Work out the finished part from the listing and answer in its coordinate system (mm). Face numbers are marked on the shaded views. A direction names the side the tool comes from. Give positions to 0.01 mm unless a question says otherwise; leave off trailing zeros. Write each loop counter-clockwise with the first axis right and the second up, starting at its lowest first coordinate (ties: lowest second). Pieces come first, ordered by that corner, then holes. Notation, with made-up numbers: (2.25, -23) - (56.25, -23) arc R25 cw to (56.25, 4) - close; hole circle Ø6 at (72, 22). An arc over 180 degrees is marked (long way). Write item = value, one per line.
from build123d import *

# Parameters (mm, degrees)
SKETCH_1_W          = 110
SKETCH_1_H          = 52.5
EXTRUDE_1_DEPTH     = 2
SKETCH_2_W          = 110
SKETCH_2_H          = 52.5
SKETCH_2_W_2        = 101.5
SKETCH_2_H_2        = 46.5
EXTRUDE_2_DEPTH     = 8.5
CUT_EXTRUDE_1_DEPTH = 3
SKETCH_5_W          = 8
SKETCH_5_H          = 46.5
CUT_EXTRUDE_2_DEPTH = 3
SKETCH_6_W          = 7
SKETCH_6_H          = 20
SKETCH_6_R          = 1.6
EXTRUDE_3_DEPTH     = 5
CHAMFER_1_SIZE      = 2


with BuildPart() as part:
    # 草图1 → 凸台-拉伸1 (new body)
    with BuildSketch(Plane.XY):
        with Locations((55, 26.25)):
            Rectangle(SKETCH_1_W, SKETCH_1_H)
    extrude(amount=EXTRUDE_1_DEPTH)

    # 草图2 → 凸台-拉伸2 (add)
    with BuildSketch(Plane.XY.offset(2)):
        with Locations((55, 26.25)):
            Rectangle(SKETCH_2_W, SKETCH_2_H)
        with Locations((55, 27.5)):
            Rectangle(SKETCH_2_W_2, SKETCH_2_H_2, mode=Mode.SUBTRACT)
    extrude(amount=EXTRUDE_2_DEPTH)

    # 草图3 → 切除-拉伸1 (cut, through all)
    with BuildSketch(Plane.XY.offset(2)):
        with BuildLine():
            Line((21.166500495, 10.551667335), (28.937295815, 6.991647804))
            ThreePointArc((28.937295815, 6.991647804), (29.429930809, 5.66601182), (28.104294825, 5.173376826))
            Line((28.104294825, 5.173376826), (20.333499505, 8.733396357))
            ThreePointArc((20.333499505, 8.733396357), (19.840864511, 10.059032341), (21.166500495, 10.551667335))
        make_face()
        with BuildLine():
            Line((91.499535297, 49.826623174), (102.166500495, 44.939786901))
            ThreePointArc((102.166500495, 44.939786901), (102.659135489, 43.614150917), (101.333499505, 43.121515923))
            Line((101.333499505, 43.121515923), (90.666534307, 48.008352196))
            ThreePointArc((90.666534307, 48.008352196), (90.173899313, 49.33398818), (91.499535297, 49.826623174))
        make_face()
        with BuildLine():
            Line((21.166500495, 16.051397639), (40.942083467, 6.991647804))
            ThreePointArc((40.942083467, 6.991647804), (41.434718462, 5.66601182), (40.109082477, 5.173376826))
            Line((40.109082477, 5.173376826), (20.333499505, 14.233126661))
            ThreePointArc((20.333499505, 14.233126661), (19.840864511, 15.558762645), (21.166500495, 16.051397639))
        make_face()
        with BuildLine():
            Line((21.166500495, 21.551127943), (52.94687112, 6.991647804))
            ThreePointArc((52.94687112, 6.991647804), (53.439506114, 5.66601182), (52.11387013, 5.173376826))
            Line((52.11387013, 5.173376826), (20.333499505, 19.732856965))
            ThreePointArc((20.333499505, 19.732856965), (19.840864511, 21.058492949), (21.166500495, 21.551127943))
        make_face()
        with BuildLine():
            Line((21.166500495, 32.550588551), (76.956446425, 6.991647804))
            ThreePointArc((76.956446425, 6.991647804), (77.449081419, 5.66601182), (76.123445435, 5.173376826))
            Line((76.123445435, 5.173376826), (20.333499505, 30.732317572))
            ThreePointArc((20.333499505, 30.732317572), (19.840864511, 32.057953556), (21.166500495, 32.550588551))
        make_face()
        with BuildLine():
            Line((21.166500495, 27.050858247), (64.951658772, 6.991647804))
            ThreePointArc((64.951658772, 6.991647804), (65.444293766, 5.66601182), (64.118657782, 5.173376826))
            Line((64.118657782, 5.173376826), (20.333499505, 25.232587268))
            ThreePointArc((20.333499505, 25.232587268), (19.840864511, 26.558223253), (21.166500495, 27.050858247))
        make_face()
        with BuildLine():
            Line((21.166500495, 38.050318854), (88.961234077, 6.991647804))
            ThreePointArc((88.961234077, 6.991647804), (89.453869071, 5.66601182), (88.128233087, 5.173376826))
            Line((88.128233087, 5.173376826), (20.333499505, 36.232047876))
            ThreePointArc((20.333499505, 36.232047876), (19.840864511, 37.55768386), (21.166500495, 38.050318854))
        make_face()
        with BuildLine():
            Line((21.166500495, 43.550049158), (100.96602173, 6.991647804))
            ThreePointArc((100.96602173, 6.991647804), (101.458656724, 5.66601182), (100.13302074, 5.173376826))
            Line((100.13302074, 5.173376826), (20.333499505, 41.73177818))
            ThreePointArc((20.333499505, 41.73177818), (19.840864511, 43.057414164), (21.166500495, 43.550049158))
        make_face()
        with BuildLine():
            Line((21.166500495, 49.049779462), (102.166500495, 11.941405078))
            ThreePointArc((102.166500495, 11.941405078), (102.659135489, 10.615769094), (101.333499505, 10.1231341))
            Line((101.333499505, 10.1231341), (20.333499505, 47.231508484))
            ThreePointArc((20.333499505, 47.231508484), (19.840864511, 48.557144468), (21.166500495, 49.049779462))
        make_face()
        with BuildLine():
            Line((31.475597035, 49.826623174), (102.166500495, 17.441135382))
            ThreePointArc((102.166500495, 17.441135382), (102.659135489, 16.115499398), (101.333499505, 15.622864403))
            Line((101.333499505, 15.622864403), (30.642596045, 48.008352196))
            ThreePointArc((30.642596045, 48.008352196), (30.149961051, 49.33398818), (31.475597035, 49.826623174))
        make_face()
        with BuildLine():
            Line((43.480384687, 49.826623174), (102.166500495, 22.940865686))
            ThreePointArc((102.166500495, 22.940865686), (102.659135489, 21.615229701), (101.333499505, 21.122594707))
            Line((101.333499505, 21.122594707), (42.647383697, 48.008352196))
            ThreePointArc((42.647383697, 48.008352196), (42.154748703, 49.33398818), (43.480384687, 49.826623174))
        make_face()
        with BuildLine():
            Line((55.48517234, 49.826623174), (102.166500495, 28.440595989))
            ThreePointArc((102.166500495, 28.440595989), (102.659135489, 27.114960005), (101.333499505, 26.622325011))
            Line((101.333499505, 26.622325011), (54.65217135, 48.008352196))
            ThreePointArc((54.65217135, 48.008352196), (54.159536356, 49.33398818), (55.48517234, 49.826623174))
        make_face()
        with BuildLine():
            Line((67.489959992, 49.826623174), (102.166500495, 33.940326293))
            ThreePointArc((102.166500495, 33.940326293), (102.659135489, 32.614690309), (101.333499505, 32.122055315))
            Line((101.333499505, 32.122055315), (66.656959002, 48.008352196))
            ThreePointArc((66.656959002, 48.008352196), (66.164324008, 49.33398818), (67.489959992, 49.826623174))
        make_face()
        with BuildLine():
            Line((79.494747645, 49.826623174), (102.166500495, 39.440056597))
            ThreePointArc((102.166500495, 39.440056597), (102.659135489, 38.114420613), (101.333499505, 37.621785619))
            Line((101.333499505, 37.621785619), (78.661746655, 48.008352196))
            ThreePointArc((78.661746655, 48.008352196), (78.16911166, 49.33398818), (79.494747645, 49.826623174))
        make_face()
    extrude(amount=-CUT_EXTRUDE_1_DEPTH, mode=Mode.SUBTRACT)

    # 草图5 → 切除-拉伸2 (cut, through all)
    with BuildSketch(Plane.XY.offset(2)):
        with Locations((8.25, 27.5)):
            Rectangle(SKETCH_5_W, SKETCH_5_H)
    extrude(amount=-CUT_EXTRUDE_2_DEPTH, mode=Mode.SUBTRACT)

    # 草图6 → 凸台-拉伸3 (add)
    with BuildSketch(Plane.XY.offset(10.5)):
        with Locations((113.5, 27.5)):
            Rectangle(SKETCH_6_W, SKETCH_6_H)
        with Locations((113.5, 32.5)):
            Circle(SKETCH_6_R, mode=Mode.SUBTRACT)
        with Locations((113.5, 22.5)):
            Circle(SKETCH_6_R, mode=Mode.SUBTRACT)
        with Locations((-3.5, 27.5)):
            Rectangle(SKETCH_6_W, SKETCH_6_H)
        with Locations((-3.5, 22.5)):
            Circle(SKETCH_6_R, mode=Mode.SUBTRACT)
        with Locations((-3.5, 32.5)):
            Circle(SKETCH_6_R, mode=Mode.SUBTRACT)
    extrude(amount=-EXTRUDE_3_DEPTH)

    # 倒角1
    chamfer_1_edges = [part.edges().sort_by_distance(p)[0] for p in [
        (110, 17.5, 8),
        (110, 37.5, 8),
        (117, 37.5, 8),
        (117, 17.5, 8),
        (0, 37.5, 8),
        (0, 17.5, 8),
        (-7, 17.5, 8),
        (-7, 37.5, 8),
    ]]
    chamfer(chamfer_1_edges, length=CHAMFER_1_SIZE)


solid = part.part
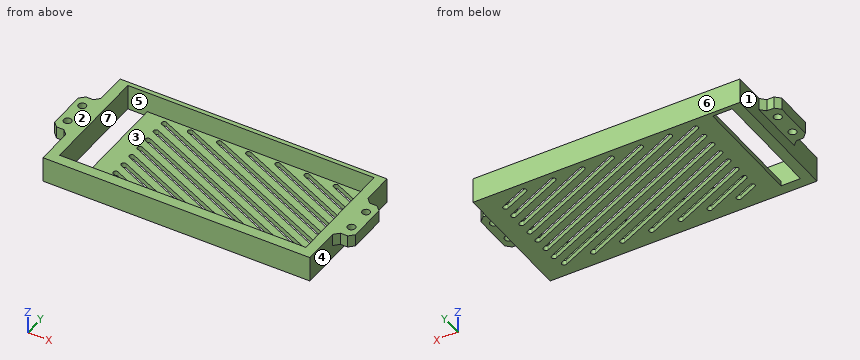
1. Find section C-C, the plane z = 3.75. Give the vertices of the cut face in (x, y), then the cut area to 3 significant figures.
Solution:
outline = (0, 0) - (110, 0) - (110, 52.5) - (0, 52.5) - close; hole (4.25, 4.25) - (105.75, 4.25) - (105.75, 50.75) - (4.25, 50.75) - close
area = 1,060 mm^2
2. For a pull along X with two mould halves and no side action, classify the marked faces 1, 2, 3 and 4 as pulls with the +X half, pulls with the -X half, needs draft (parallel to the pull), parting line crosses it, or undercut.
Solution:
face_1 = pulls with the -X half
face_2 = needs draft
face_3 = undercut
face_4 = pulls with the +X half
3. Straight lines are drawn through the part: line 1 (Y direction, x = 113.5, z = 9); line 2 (X direction, y = 40.5, z = 9); line 3 (Y direction, x = 82.5, z = 4.75). For each, find the intervals that lie inside material, in ascending order.
Solution:
line_1 = 17.5 to 20.9, 24.1 to 30.9, 34.1 to 37.5
line_2 = 0 to 4.25, 105.75 to 110
line_3 = 0 to 4.25, 50.75 to 52.5
4. A tool of negligible diameter and unlimited length cuts with its end or side. For the marked faces 5, 6 and 7, from which of +Z, -Z, +X, -X, +Y, -Y can it reach the whole face along a straight path? Write none if from no direction.
Solution:
face_5 = +Z
face_6 = +Z, -Z, +X, -X, +Y
face_7 = +Z, -Z
5. Find section A-A, the plane x = 113.5. Give the vertices of the cut face in (y, z).
Solution:
outline = (17.5, 5.5) - (20.9, 5.5) - (20.9, 10.5) - (17.5, 10.5) - close; (24.1, 5.5) - (30.9, 5.5) - (30.9, 10.5) - (24.1, 10.5) - close; (34.1, 5.5) - (37.5, 5.5) - (37.5, 10.5) - (34.1, 10.5) - close
6. Find section B-B, the plane z = 9.25. Give the vertices of the cut face in (x, y), then the cut area to 3 significant figures.
Solution:
outline = (-7, 19.5) - (-5, 17.5) - (-2, 17.5) - (0, 15.5) - (0, 0) - (110, 0) - (110, 15.5) - (112, 17.5) - (115, 17.5) - (117, 19.5) - (117, 35.5) - (115, 37.5) - (112, 37.5) - (110, 39.5) - (110, 52.5) - (0, 52.5) - (0, 39.5) - (-2, 37.5) - (-5, 37.5) - (-7, 35.5) - close; hole circle Ø3.2 at (-3.5, 22.5); hole circle Ø3.2 at (-3.5, 32.5); hole (4.25, 4.25) - (105.75, 4.25) - (105.75, 50.75) - (4.25, 50.75) - close; hole circle Ø3.2 at (113.5, 22.5); hole circle Ø3.2 at (113.5, 32.5)
area = 1,300 mm^2
7. Given pin 1 (12 mm diameter, centred on x = 11, y = 26, fed in from +Z); pin 2 (1.5 mm diameter, centred on x = -4, z = 7, fed in from -Y); pin 3 (2.5 mm diameter, centred on x = -3, z = 7.5, fed in from +Y), each flat-ended and moving along its own axis, determine where each tip first touches the part or whether it passes through.
Solution:
pin_1 = 2
pin_2 = 17.5
pin_3 = 37.75
